CAD build for the part. Positions are in the model's coordinates, mm. A direction names the side the tool comes from. Give positions to 0.01 mm unless a question says otherwise; leave off trailing zeros. Loops run counter-clockwise (first coordinate to the right, second up) from the corner with the lowest first, then second, coordinate; pieces in that order, holes last. Notation, with made-up numbers: (-29, 76.5) -> (12, 76.5) arc R5 ccw to (12, 81.5) -> close; hole circle Ø7 at (31, 80.25). An arc over 180 degrees is marked (long way). Use one line per item in the form item = value.
Autodesk Inventor part; units mm, degrees
ref_plane "YZ Plane" through (0, 0, 0) normal (1, 0, 0) x (0, 1, 0)
ref_plane "XZ Plane" through (0, 0, 0) normal (0, 1, 0) x (-1, 0, 0)
ref_plane "XY Plane" through (0, 0, 0) normal (0, 0, 1) x (1, 0, 0)
sketch "Skizze1" plane through (0, 0, 0) normal (0, 0, 1) x (1, 0, 0)
  line L0 (-18, 0) -> (3, 0)
  line L1 (0, -0.8) -> (0, 4.8)
  line L2 (0, 2) -> (-7.5, 2)
  line L3 (-7.5, 2) -> (-7.5, 4)
  line L4 (-7.5, 4) -> (-9, 4)
  line L5 (-9, 4) -> (-9, 2.5)
  line L6 (-9, 2.5) -> (-15, 2.5)
  line L7 (-15, 2.5) -> (-15, 0)
  line L8 (-15, 0) -> (0, 0)
  line L9 (0, 0) -> (0, 2)
  dimension "d0" = 4
  dimension "d1" = 8
  dimension "d2" = 5
  dimension "d3" = 7.5
  dimension "d4" = 1.5
  dimension "d5" = 6
revolve "Umdrehung1" add sketch "Skizze1" angle 360 about axis through (-10, 0, 0) along (1, 0, 0)
sketch "Skizze2" plane through (-15, 0, 0) normal (-1, 0, 0) x (0, 0, 1)
  circle A0 centre (0, 0) radius 2.5
  line L0 (1.5, 2) -> (1.5, -2)
  dimension "d7" = 1
extrude "Extrusion1" cut sketch "Skizze2" against normal blind 4 contours A0 L0 picked at (1.6398, 0.534)
sketch "Skizze3" plane through (0, 0, 0) normal (0, 1, 0) x (-1, 0, 0)
  line L0 (1.5, 2) -> (1, 2)
  line L1 (1, 2) -> (1, 1.9)
  line L2 (1, 1.9) -> (1.5, 1.9)
  line L3 (1.5, 1.9) -> (1.5, 2)
  line L4 (2.4, 0) -> (-0.4, 0)
  line L5 (0, -0.4) -> (0, 2.4)
  point P0 (0, 0)
  dimension "d10" = 3.8
  dimension "d11" = 1.5
  dimension "d12" = 0.5
  dimension "d13" = 4
revolve "Umdrehung2" cut sketch "Skizze3" angle 360 about axis through (-10, 0, 0) along (1, 0, 0)
chamfer "Fase1" distance 0.5 angle 45 1 edges at (0, -2, 0)
properties part number "13_1087_016"
1. Mould opens along X. For faces 1 (the cylindrical face through (-1.25, 0.08, -1.9)), 2 (the flat face through (-7.5, -2, -1)), 3 (the cylindrical face through (-5, 0, 2)) say: pulls with the +X half, pulls with the -X half, needs draft (parallel to the pull), parting line crosses it, or undercut.
Result sheet:
face_1 = undercut
face_2 = pulls with the +X half
face_3 = needs draft
2. Tool access for faces 4 (the flat face through (-9, 2, 2)), 5 (the flat face through (-11, 0, 2)), 6 (the cylindrical face through (-0.754, -0.434, 1.952)): list every direction of +Z, -Z, +X, -X, +Y, -Y with a clear straight run to the whole face (end or side of a thin tool).
Result sheet:
face_4 = -X
face_5 = +Z, -X, +Y, -Y
face_6 = +X
3. Cut at A-A, the plane z = 0. Write the cut outline in (x, y), then the cut area to 4 significant figures.
Result sheet:
outline = (-15, -2.5) -> (-9, -2.5) -> (-9, -4) -> (-7.5, -4) -> (-7.5, -2) -> (-1.5, -2) -> (-1.5, -1.9) -> (-1, -1.9) -> (-1, -2) -> (-0.5, -2) -> (0, -1.5) -> (0, 1.5) -> (-0.5, 2) -> (-1, 2) -> (-1, 1.9) -> (-1.5, 1.9) -> (-1.5, 2) -> (-7.5, 2) -> (-7.5, 4) -> (-9, 4) -> (-9, 2.5) -> (-15, 2.5) -> close
area = 71.65 mm^2
4. Cut at B-B, the plane y = 0. Write the cut outline in (x, z).
Result sheet:
outline = (-15, -2.5) -> (-9, -2.5) -> (-9, -4) -> (-7.5, -4) -> (-7.5, -2) -> (-1.5, -2) -> (-1.5, -1.9) -> (-1, -1.9) -> (-1, -2) -> (-0.5, -2) -> (0, -1.5) -> (0, 1.5) -> (-0.5, 2) -> (-1, 2) -> (-1, 1.9) -> (-1.5, 1.9) -> (-1.5, 2) -> (-7.5, 2) -> (-7.5, 4) -> (-9, 4) -> (-9, 2.5) -> (-11, 2.5) -> (-11, 1.5) -> (-15, 1.5) -> close
5. Cut at C-C, the plane x = -8.5. Write the cut outline in (y, z).
Result sheet:
outline = circle Ø8 at (0, 0)
6. Cut at D-D, the plane x = -2.25. Write the cut outline in (y, z).
Result sheet:
outline = circle Ø4 at (0, 0)
7. Drill centre lines: line 1 (X direction, y = 0, z = 3.5); line 2 (X direction, y = 1.75, z = -1.25); line 3 (Y direction, x = -11, z = -1.5). Where is each one in solid material? Low to high.
Result sheet:
line_1 = -9 to -7.5
line_2 = -15 to -7.5
line_3 = -2 to 2
8. Drop flat-ended pins along their axis: P1, Ø2, axis at x = -8.5, z = 2.5, coming from the +Y side; P2, Ø4, axis at x = -10, y = 0, coming from the +Z side; P3, Ø0.8, axis at y = 0.5, z = 2, coming from the -X side. Give the stop position or say it passes through.
Result sheet:
P1 = 3.71
P2 = 4
P3 = -11
